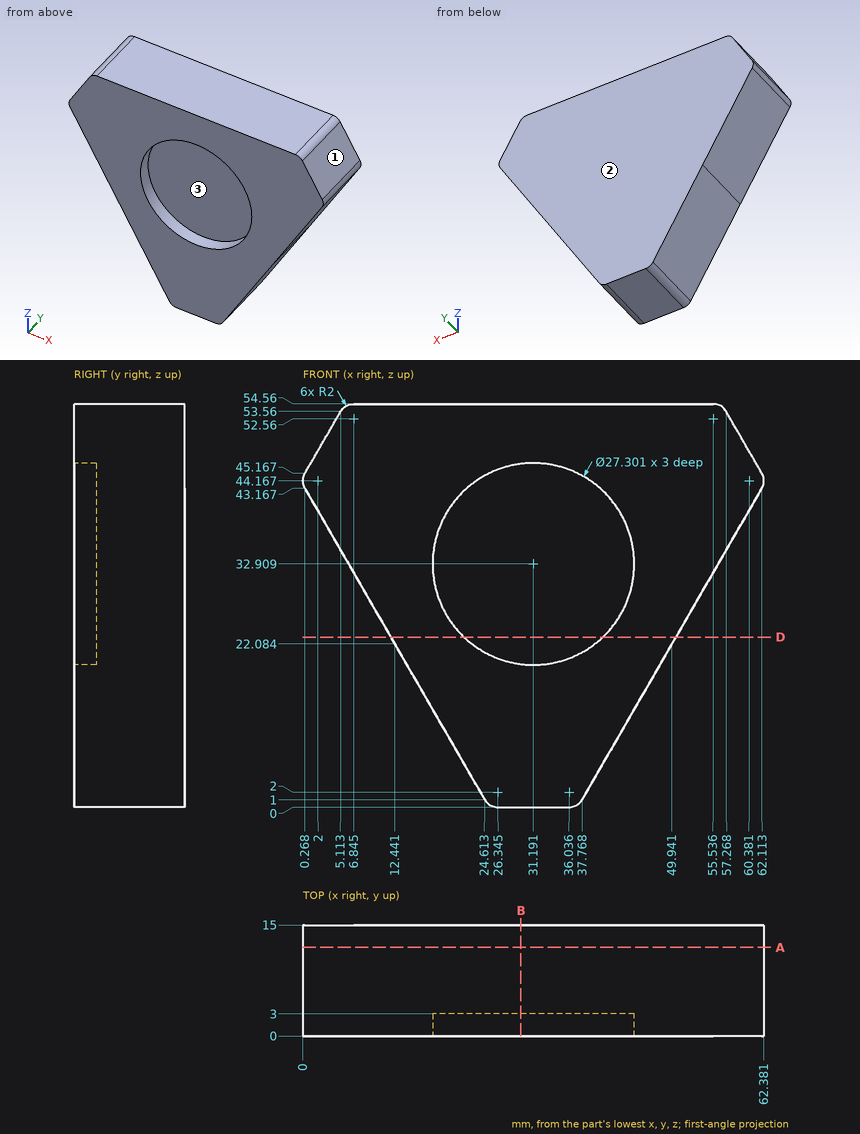
Part print with two shaded views. Sizes in mm from the minimum x, y, z corner. Round coordinates to 2 decimals unless told otherwise and drop trailing zeros. Order: outer loops, then holes, each group sorted by start corner. A loop starts at its lowest first (then second) coordinate and runs counter-clockwise, first axis right, second up. Notation, with made-up numbers: (-24.75, 84) -> (-15.75, 84) arc R12 cw to (-15.75, 89) -> close; hole circle Ø2 at (8, 31). An arc over 180 degrees is marked (long way). Use one line per item in the form item = value.
Item 1: Cut at B-B, the plane x = 29.5. Write the cut outline in (y, z) (1 decimal), and give its area (3 significant figures).
Returned:
outline = (0, 0) -> (15, 0) -> (15, 54.6) -> (0, 54.6) -> (0, 46.5) -> (3, 46.5) -> (3, 19.4) -> (0, 19.4) -> close
area = 737 mm^2
Item 2: Pull direction X, two halves, no side cores. Call the marked faces 1, 2 and 3: released by +X, released by -X, zero draft, split by the parting line, or undercut.
Returned:
face_1 = released by +X
face_2 = zero draft
face_3 = undercut
Item 3: Drill centre lines: line 1 (Z direction, x = 7, y = 12.5) (1 decimal); line 2 (X direction, y = 1.75, z = 8); line 3 (Z direction, x = 21, y = 11.75) (1 decimal). Where is each one in solid material? Low to high.
Returned:
line_1 = 31.5 to 54.6
line_2 = 20.57 to 41.81
line_3 = 7.3 to 54.6
Item 4: Flat gauge pins, fed straight in: pin 1 Ø4 at (x, y) = (40.5, 4.5) entering from -Z; pin 2 Ø3 at (y, z) = (3.5, 21.5) entering from -X; pin 3 Ø1 at (x, y) = (25, 3) entering from -Z; pin 4 Ø13.5 at (x, z) = (36, 38) entering from -Y. Where does each tip first touch, or does it go through?
Returned:
pin_1 = 2.27
pin_2 = 11.91
pin_3 = 0.19
pin_4 = 0
Item 5: Cut at D-D, the plane z = 23. Write the cut outline in (x, y).
Returned:
outline = (11.91, 0) -> (21.8, 0) -> (21.8, 3) -> (40.58, 3) -> (40.58, 0) -> (50.47, 0) -> (50.47, 15) -> (11.91, 15) -> close
Item 6: Cut at A-A, the plane y = 12. Write the cut outline in (x, z) (1 decimal).
Returned:
outline = (0.3, 43.2) -> (24.6, 1) arc R2 ccw to (26.3, 0) -> (36, 0) arc R2 ccw to (37.8, 1) -> (62.1, 43.2) arc R2 ccw to (62.1, 45.2) -> (57.3, 53.6) arc R2 ccw to (55.5, 54.6) -> (6.8, 54.6) arc R2 ccw to (5.1, 53.6) -> (0.3, 45.2) arc R2 ccw to start
